```python
from build123d import *

# Parameters (mm, degrees)
BOSS_EXTRUDE1_DEPTH = 42
SKETCH3_R           = 3
CUT_EXTRUDE1_DEPTH  = 14.120795661
SKETCH4_R           = 14
CUT_EXTRUDE3_DEPTH  = 3
SKETCH5_R           = 9
CUT_EXTRUDE4_DEPTH  = 5
SKETCH6_R           = 1.7
CUT_EXTRUDE5_DEPTH  = 11.41
SKETCH7_R           = 1.7
CUT_EXTRUDE6_DEPTH  = 41.679003175
BOSS_EXTRUDE2_DEPTH = 2
BOSS_EXTRUDE3_DEPTH = 2


with BuildPart() as part:
    # Sketch1 → Boss-Extrude1 (new body)
    with BuildSketch(Plane.XY):
        Polygon((0, 0), (42, 0), (42, 75.879204339), (83.679003175, 75.879204339), (83.679003175, -14.120795661), (42, -14.120795661), (0, -14.120795661), align=None)
    extrude(amount=BOSS_EXTRUDE1_DEPTH)

    # Sketch3 → Cut-Extrude1 (cut)
    with BuildSketch(Plane(origin=(0, 0, 0), x_dir=(1, 0, 0), z_dir=(0, 1, 0))):
        with Locations(Location((21, -21, 0), (0, 0, 270))):
            Circle(SKETCH3_R)
    extrude(amount=-CUT_EXTRUDE1_DEPTH, mode=Mode.SUBTRACT)

    # Sketch4 → Cut-Extrude3 (cut)
    with BuildSketch(Plane(origin=(0, 0, 0), x_dir=(1, 0, 0), z_dir=(0, 1, 0))):
        with Locations(Location((21, -21, 0), (0, 0, 270))):
            Circle(SKETCH4_R)
    extrude(amount=-CUT_EXTRUDE3_DEPTH, mode=Mode.SUBTRACT)

    # Sketch5 → Cut-Extrude4 (cut)
    with BuildSketch(Plane(origin=(0, 0, 0), x_dir=(1, 0, 0), z_dir=(0, 1, 0))):
        with Locations(Location((21, -21, 0), (0, 0, 270))):
            Circle(SKETCH5_R)
    extrude(amount=-CUT_EXTRUDE4_DEPTH, mode=Mode.SUBTRACT)

    # Sketch6 → Cut-Extrude5 (cut)
    with BuildSketch(Plane(origin=(0, -3, 0), x_dir=(1, 0, 0), z_dir=(0, 1, 0))):
        with Locations(Location((21, -10, 0), (0, 0, 270))):
            Circle(SKETCH6_R)
        with Locations(Location((32, -21, 0), (0, 0, 270))):
            Circle(SKETCH6_R)
        with Locations(Location((21, -32, 0), (0, 0, 270))):
            Circle(SKETCH6_R)
        with Locations(Location((10, -21, 0), (0, 0, 270))):
            Circle(SKETCH6_R)
    extrude(amount=-CUT_EXTRUDE5_DEPTH, mode=Mode.SUBTRACT)

    # Sketch7 → Cut-Extrude6 (cut)
    with BuildSketch(Plane.ZY.offset(-42)):
        with Locations((10.5, 56.654204339)):
            Circle(SKETCH7_R)
        with Locations((31.5, 56.654204339)):
            Circle(SKETCH7_R)
        with Locations((10.5, 18.71460217)):
            Circle(SKETCH7_R)
        with Locations((31.5, 18.71460217)):
            Circle(SKETCH7_R)
    extrude(amount=-CUT_EXTRUDE6_DEPTH, mode=Mode.SUBTRACT)

    # Sketch8 → Boss-Extrude2 (add)
    with BuildSketch(Plane.XY.offset(42)):
        Polygon((42, 37.93960217), (21, 0), (42, 0), align=None)
    extrude(amount=-BOSS_EXTRUDE2_DEPTH)

    # Sketch9 → Boss-Extrude3 (add)
    with BuildSketch(Plane(origin=(0, 0, 0), x_dir=(-1, 0, 0), z_dir=(0, 0, -1))):
        Polygon((-42, 37.93960217), (-21, 0), (-42, 0), align=None)
    extrude(amount=-BOSS_EXTRUDE3_DEPTH)


solid = part.part
```
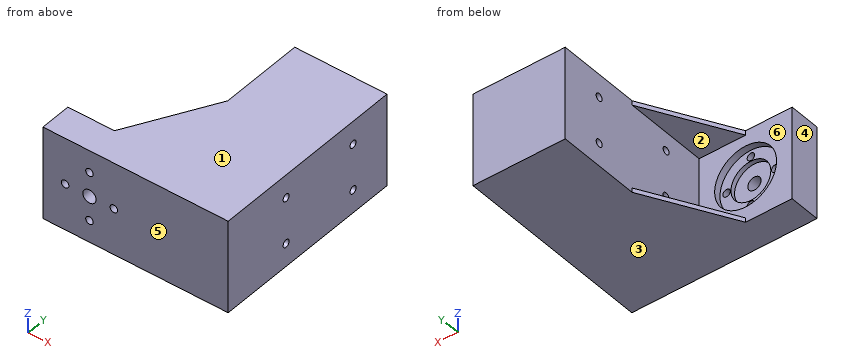
Verification items for the finished model (mm, model axes). Face numbers are marked on the shaded views. A direction names the side the tool comes from. Give positions to 0.01 mm unless a question says otherwise; leave off trailing zeros. Order: outer loops, then holes, each group sorted by start corner. A loop starts at its lowest first (then second) coordinate and runs counter-clockwise, first axis right, second up. Notation, with made-up numbers: M 33,14 L 51,14 A6 ccw 51,18 Z; hole C 13,-12.75 d8. An arc over 180 degrees is marked long. Answer in a Markdown table with one row per item. Add a question column.
Item 1: Gauge pin test, flat ends, axial feed: pin 1 (4.5 mm diameter, centred on y = 56.65, z = 31.5, fed in from -X); pin 2 (7 mm diameter, centred on x = 21, z = 21, fed in from +Y); pin 3 (14 mm diameter, centred on x = 18, z = 17.5, fed in from +Y); pin 4 (10 mm diameter, centred on x = 20, y = 15, fed in from -Z). Record the tip position at first contact, or that the pin passes through.
Item 2: Mould release check, pull along Z, two halves, no side actions. Record for the marked faces 1, 2, 3 and 4: released by +Z, released by -Z, zero draft, split by the parting line, or undercut.
Item 3: Scan lines: probe 1 along Y at (x, z) = (60, 31.5); probe 2 along X at (y, z) = (-3.5, 21); probe 3 along X at (y, z) = (-8, 22). Record each from-to range of solid material in increasing order. Write a range as from..to.
Item 4: Section check C-C, the plane z = 10.5. Enter the section's corners in (x, y).
Item 5: Section check D-D, the plane y = 45.5. Enter the section's corners in (x, z), and give its area (3 significant figures).
Item 6: Section check A-A, the plane z = 4. Enter the section's corners in (x, y), and give its area (3 significant figures).
Item 7: Tool access check on the marked faces 5 and 6. Record the directions out of +Z, -Z, +X, -X, +Y, -Y that give a thin tool (end or side, any length) a straight path to the whole face; none if there is none.
Item 8: Section check B-B, the plane x = 32. Enter the section's corners in (y, z).
Filled sheet:
| question | item | result |
|---|---|---|
| 1 | pin 1 | stops at x = 42 |
| 1 | pin 2 | stops at y = -5 |
| 1 | pin 3 | stops at y = -3 |
| 1 | pin 4 | passes through |
| 2 | face 1 | released by +Z |
| 2 | face 2 | undercut |
| 2 | face 3 | released by -Z |
| 2 | face 4 | zero draft |
| 3 | probe 1 | y = -14.12..17.01, 20.41..54.95, 58.35..75.88 |
| 3 | probe 2 | x = 0..8.3, 11.7..12, 30..30.3, 33.7..83.68 |
| 3 | probe 3 | x = 0..8.63, 11.37..18.17, 23.83..30.63, 33.37..83.68 |
| 4 | outline | M 0,-14.12 L 19.38,-14.12 L 19.38,-3 L 11.74,-3 L 11.74,0 L 0,0 Z; M 22.62,-14.12 L 83.68,-14.12 L 83.68,17.01 L 42,17.01 L 42,0 L 30.26,0 L 30.26,-3 L 22.62,-3 Z; M 42,20.41 L 83.68,20.41 L 83.68,54.95 L 42,54.95 Z; M 42,58.35 L 83.68,58.35 L 83.68,75.88 L 42,75.88 Z |
| 5 | outline | M 42,0 L 83.68,0 L 83.68,42 L 42,42 Z |
| 5 | area | 1,750 mm^2 |
| 6 | outline | M 0,-14.12 L 83.68,-14.12 L 83.68,75.88 L 42,75.88 L 42,0 L 0,0 Z |
| 6 | area | 4,340 mm^2 |
| 7 | face 5 | +Z, -Z, +X, -X, -Y |
| 7 | face 6 | -X, +Y |
| 8 | outline | M -14.12,0 L 19.87,0 L 19.87,2 L 0,2 L 0,12.34 L -3,12.34 L -3,19.3 L -14.12,19.3 Z; M -14.12,22.7 L -3,22.7 L -3,29.66 L 0,29.66 L 0,40 L 19.87,40 L 19.87,42 L -14.12,42 Z |
